Autodesk Inventor part; units mm, degrees
ref_plane "Work Plane1" through (0, 406.4, 0) normal (0, 1, 0) x (-1, 0, 0)
ref_plane "YZ Plane" through (0, 0, 0) normal (1, 0, 0) x (0, 1, 0)
ref_plane "XY Plane" through (0, 0, 0) normal (0, 0, 1) x (1, 0, 0)
sketch "Sketch1" plane through (0, 0, 0) normal (0, 0, 1) x (1, 0, 0)
  circle A0 centre (0, 0) radius 406.4
  circle A1 centre (0, 0) radius 393.7
  dimension "d0" = 812.8
  dimension "d1" = 787.4
extrude "Extrusion1" add sketch "Sketch1" along normal blind 153.4
chamfer "Chamfer1" distance 11.1125 angle 37.5 1 edges at (-406.4, 0, 0) measured on face at (401.8367, 9.4497, 0)
chamfer "Chamfer2" distance 11.1125 angle 40 1 edges at (-393.7, 0, 153.4) measured on face at (401.8367, 9.4497, 153.4)
ref_plane "Work Plane1" through (0, 406.4, 0) normal (0, 1, 0) x (-1, 0, 0)
sketch "Sketch2" plane through (0, 406.4, 0) normal (0, 1, 0) x (-1, 0, 0)
  point P0 (0, 0)
  point P1 (0, 57.9438)
  dimension "d10" = 57.9438
hole "Hole1" at (0, 406.4, 57.9438) direction (0, -1, 0) diameter 22.6314 depth 23.114 tip angle 118
pattern_circular "Circular Pattern1" count 2 over 360 about axis through (0, 0, -10) along (0, 0, 1) of "Hole1"
equation "\"d7\" = d4"
properties part number "A1-19027-300-01 32in pipe" material "Steel, Mild"
The listing builds one solid part. Answer for the finished solid, in the listing's coordinates (mm). Round coordinates to 2 decimals unless told otherwise and drop trailing zeros. Loops run counter-clockwise (first coordinate to the right, second up) from the corner with the lowest first, then second, coordinate; pieces in that order, holes last. Notation, with made-up numbers: (-4, 85) -> (12, 85) arc R19 cw to (12, 105) -> close; hole circle Ø3 at (17.25, 62). An arc over 180 degrees is marked (long way). Use one line per item in the form item = value.
1. The part is cut by section C-C on z = 93.5. Determine the outline of the cut face in (x, y).
Answer key:
outline = circle Ø812.8 at (0, 0); hole circle Ø787.4 at (0, 0)
2. The part is cut by section B-B on x = 0. Determine the outline of the cut face in (y, z).
Answer key:
outline = (-406.4, 8.53) -> (-395.29, 0) -> (-393.7, 0) -> (-393.7, 46.63) -> (-406.4, 46.63) -> close; (-406.4, 69.26) -> (-393.7, 69.26) -> (-393.7, 144.08) -> (-404.81, 153.4) -> (-406.4, 153.4) -> close; (393.7, 0) -> (395.29, 0) -> (406.4, 8.53) -> (406.4, 46.63) -> (393.7, 46.63) -> close; (393.7, 69.26) -> (406.4, 69.26) -> (406.4, 153.4) -> (404.81, 153.4) -> (393.7, 144.08) -> close
3. Find the intervals of material crossed by probe 1 along Y at (x, z) = (0, 46); probe 2 along Z at (x, y) = (0, 400); probe 3 along X at (y, z) = (-83, 76.5), in increasing order. Write a range as [from, to].
Answer key:
probe_1 = [-406.4, -393.7], [393.7, 406.4]
probe_2 = [3.62, 46.63], [69.26, 149.36]
probe_3 = [-397.83, -384.85], [384.85, 397.83]
4. For a pull along X with two mould halves and no side action, classify faces 1 (the cylindrical face through (-4.33, -399.88, 68.4)), 2 (the conical face through (-51.55, 392.61, 0.53)) as released by +X, released by -X, zero draft, split by the parting line, or undercut.
Answer key:
face_1 = undercut
face_2 = split by the parting line
5. The part is cut by section A-A on y = 0. Determine the outline of the cut face in (x, z), and give its area (3 significant figures).
Answer key:
outline = (-406.4, 8.53) -> (-395.29, 0) -> (-393.7, 0) -> (-393.7, 144.08) -> (-404.81, 153.4) -> (-406.4, 153.4) -> close; (393.7, 0) -> (395.29, 0) -> (406.4, 8.53) -> (406.4, 153.4) -> (404.81, 153.4) -> (393.7, 144.08) -> close
area = 3,700 mm²
6. Flat-ended cylindrical pins translate along their axes: pin 1 Ø10 at (y, z) = (-157, 138) entering from +X; pin 2 Ø1 at (x, z) = (185.5, 50.5) entering from +Y; pin 3 Ø3 at (y, z) = (-200.5, 98) entering from +X. Find the tip coordinate at first contact, or state that the pin passes through.
Answer key:
pin_1 = 376.9
pin_2 = 361.85
pin_3 = 354.34
